Work out the finished part from the listing and answer in its coordinate system (mm). A direction names the side the tool comes from. Round coordinates to 2 decimals unless told otherwise and drop trailing zeros. Loops run counter-clockwise (first coordinate to the right, second up) from the corner with the lowest first, then second, coordinate; pieces in that order, holes last.
```python
from build123d import *

# Parameters (mm, degrees)
SKETCH_1_R          = 2.1
SKETCH_1_R_2        = 2
SKETCH_1_R_3        = 9.52
SKETCH_1_R_4        = 2.05
SKETCH_1_R_5        = 1.65
EXTRUDE_1_DEPTH     = 2
SKETCH_3_W          = 52.726125437
SKETCH_3_H          = 0.98
EXTRUDE_2_DEPTH     = 2
SKETCH_2_R          = 2.05
SKETCH_2_R_2        = 3.1
SKETCH_2_W          = 32.809844138
SKETCH_2_H          = 42
CUT_EXTRUDE_1_DEPTH = 4
FILLET_1_R          = 2
FILLET_2_R          = 5


with BuildPart() as part:
    # 草图1 → 凸台-拉伸1 (new body)
    with BuildSketch(Plane.XY):
        with BuildLine():
            Line((-1.457142857, 39.854285714), (328.542857143, 39.854285714))
            Line((328.542857143, 39.854285714), (334.49569518, 22.070579719))
            ThreePointArc((334.49569518, 22.070579719), (346.78998397, 13.855798581), (351.542857143, -0.145714286))
            Line((351.542857143, -0.145714286), (356.542857143, -22.235997541))
            Line((356.542857143, -22.235997541), (356.542857143, -40.145714286))
            Line((356.542857143, -40.145714286), (328.542857143, -40.145714286))
            Line((328.542857143, -40.145714286), (126.194823947, -40.145714286))
            Line((126.194823947, -40.145714286), (113.608549915, -61.445714286))
            Line((113.608549915, -61.445714286), (101.341389716, -61.445714286))
            Line((101.341389716, -61.445714286), (93.462833584, -40.145714286))
            Line((93.462833584, -40.145714286), (-1.457142857, -40.145714286))
            ThreePointArc((-1.457142857, -40.145714286), (-41.457142857, -0.145714286), (-1.457142857, 39.854285714))
        make_face()
        with Locations((-1.457142857, -23.895714286)):
            Circle(SKETCH_1_R, mode=Mode.SUBTRACT)
        with Locations((18.028428728, -11.395714286)):
            Circle(SKETCH_1_R, mode=Mode.SUBTRACT)
        with Locations((-1.457142857, -0.145714286)):
            Circle(SKETCH_1_R_2, mode=Mode.SUBTRACT)
        with Locations((328.542857143, -0.145714286)):
            Circle(SKETCH_1_R_3, mode=Mode.SUBTRACT)
        with Locations((288.542857143, -0.145714286)):
            Circle(SKETCH_1_R_4, mode=Mode.SUBTRACT)
        with Locations((238.542857143, 16.354285714)):
            Circle(SKETCH_1_R_4, mode=Mode.SUBTRACT)
        with Locations(Location((238.542857143, -16.645714286, 0), (0, 0, 180))):
            Circle(SKETCH_1_R_4, mode=Mode.SUBTRACT)
        with Locations((-20.942714442, -11.395714286)):
            Circle(SKETCH_1_R, mode=Mode.SUBTRACT)
        with Locations((-22.025246197, 11.729285714)):
            Circle(SKETCH_1_R, mode=Mode.SUBTRACT)
        with Locations((-1.457142857, 22.354285714)):
            Circle(SKETCH_1_R, mode=Mode.SUBTRACT)
        with Locations((19.110960483, 11.729285714)):
            Circle(SKETCH_1_R, mode=Mode.SUBTRACT)
        with Locations((7.042857143, -8.645714286)):
            Circle(SKETCH_1_R_5, mode=Mode.SUBTRACT)
        with Locations((-9.957142857, -8.645714286)):
            Circle(SKETCH_1_R_5, mode=Mode.SUBTRACT)
        with Locations((-9.957142857, 8.354285714)):
            Circle(SKETCH_1_R_5, mode=Mode.SUBTRACT)
        with Locations((7.042857143, 8.354285714)):
            Circle(SKETCH_1_R_5, mode=Mode.SUBTRACT)
    extrude(amount=EXTRUDE_1_DEPTH)

    # 草图3 → 凸台-拉伸2 (add)
    with BuildSketch(Plane.XY.offset(2)):
        with Locations((24.905919862, 40.344285714)):
            Rectangle(SKETCH_3_W, SKETCH_3_H)
    extrude(amount=-EXTRUDE_2_DEPTH)

    # 草图2 → 切除-拉伸1 (cut)
    with BuildSketch(Plane.XY.offset(2)):
        with Locations((18.542857143, 33.854285714)):
            Circle(SKETCH_2_R)
        with Locations((108.542857143, 33.854285714)):
            Circle(SKETCH_2_R)
        with Locations((198.542857143, 33.854285714)):
            Circle(SKETCH_2_R)
        with Locations((108.542857143, -34.145714286)):
            Circle(SKETCH_2_R)
        with Locations((198.542857143, -34.145714286)):
            Circle(SKETCH_2_R)
        with Locations((288.542857143, -34.145714286)):
            Circle(SKETCH_2_R_2)
        with Locations((18.542857143, -34.145714286)):
            Circle(SKETCH_2_R)
        with Locations((288.542857143, 33.854285714)):
            Circle(SKETCH_2_R_2)
        Polygon((31.542857143, -21.145714286), (104.183898028, -21.145714286), (159.772133322, 20.854285714), (31.542857143, 20.854285714), align=None)
        Polygon((148.123425102, -21.145714286), (203.711660396, 20.854285714), (233.542857143, 20.854285714), (233.542857143, -21.145714286), align=None)
        with Locations((259.947779212, -0.145714286)):
            Rectangle(SKETCH_2_W, SKETCH_2_H)
    extrude(amount=-CUT_EXTRUDE_1_DEPTH, mode=Mode.SUBTRACT)

    # 圆角1
    fillet_1_edges = [part.edges().sort_by_distance(p)[0] for p in [
        (31.542857143, -21.145714286, 1),
        (31.542857143, 20.854285714, 1),
        (159.772133322, 20.854285714, 1),
        (104.183898028, -21.145714286, 1),
        (243.542857143, 20.854285714, 1),
        (276.352701281, 20.854285714, 1),
        (276.352701281, -21.145714286, 1),
        (243.542857143, -21.145714286, 1),
        (203.711660396, 20.854285714, 1),
        (233.542857143, 20.854285714, 1),
        (233.542857143, -21.145714286, 1),
        (148.123425102, -21.145714286, 1),
    ]]
    fillet(fillet_1_edges, radius=FILLET_1_R)

    # 圆角2
    fillet_2_edges = [part.edges().sort_by_distance(p)[0] for p in [
        (356.542857143, -40.145714286, 1),
    ]]
    fillet(fillet_2_edges, radius=FILLET_2_R)


solid = part.part
```
1. Which of the six approach directions +Z, -Z, +X, -X, +Y, -Y give full straight-line access (tool end or side, diameter ignored) to faces 4 (the face through (155, 2, 2)), 5 (the face through (177.7, 1.2, 1))?
Answer key:
face 4: +Z, +X, -X, +Y, -Y
face 5: +Z, -Z
2. Determine the mould class of faces 1 (the face through (97.457, -50.945, 0.986)), 2 (the face through (291.406, -35.333, 1.014)), 3 (the face through (-41.447, -1.025, 0.986)) for opening direction Y: +Y half, -Y half, draft (parallel to the pull), parting line (faces both ways), or undercut.
Answer key:
face 1: -Y half
face 2: undercut
face 3: parting line
3. Find section C-C (y = -46.5). Write down the section's boundary in (x, z).
Answer key:
outline: (95.81, 0) - (122.44, 0) - (122.44, 2) - (95.81, 2) - close
4. Find section B-B (z = 0.6). Give the number of separate pieces and of enclosed holes in the cut face, then the cut area to 3 significant figures.
Answer key:
separate pieces: 1
enclosed holes: 26
area: 22,400 mm2
5. Consider probe 1 along Y at (x, z) = (265, 0.3); probe 2 along Y at (x, z) = (47, 0.25); probe 3 along X at (y, z) = (-15, 0.55). Determine where each line is inside the solid, lowest interval first.
Answer key:
probe 1: y = -40.15 to -21.15, 20.85 to 39.85
probe 2: y = -40.15 to -21.15, 20.85 to 40.83
probe 3: x = -38.6 to 31.54, 112.32 to 156.26, 233.54 to 237.32, 239.77 to 243.54, 276.35 to 354.91
6. Find section A-A (x = 209.5). Write down the section's boundary in (y, z).
Answer key:
outline: (-40.15, 0) - (-21.15, 0) - (-21.15, 2) - (-40.15, 2) - close; (20.85, 0) - (39.85, 0) - (39.85, 2) - (20.85, 2) - close
7. Given pin 1 (0.6 mm diameter, centred on x = 249, z = 1.5, fed in from +Y); pin 2 (1 mm diameter, centred on x = 68.5, z = 1, fed in from -Y); pin 3 (1 mm diameter, centred on y = 5.5, z = 1.5, fed in from +X), each flat-ended and moving along its own axis, determine where each tip first touches the part or whether it passes through.
Answer key:
pin 1: stops at y = 39.85
pin 2: stops at y = -40.15
pin 3: stops at x = 350.96
